Read the model definition and answer for the solid it produces. Units are mm, in the model's axes. A direction names the side the tool comes from. Coordinates: 2 decimals unless noted, no trailing zeros. Order: outer loops, then holes, each group sorted by start corner. A loop starts at its lowest first (then second) coordinate and runs counter-clockwise, first axis right, second up. Notation, with made-up numbers: (2, 62) -> (53, 62) arc R16 cw to (53, 70) -> close; hole circle Ø9 at (-14, -14.5). An arc over 180 degrees is marked (long way). Use CSV: the item, a comma, the result in double quotes.
```python
from build123d import *

# Parameters (mm, degrees)
F0_R     = 12.7
F1_DEPTH = 152.4
F2_R     = 76.19999
F3_R     = 38.1
F4_DEPTH = 41.7364233324
F7_DEPTH = 96.9898923586
F8_DEPTH = 152.401


# Not quite as in the source:
# - a fillet or chamfer is up to 0.001 mm smaller than in the source, because OpenCascade refuses the exact size


with BuildPart() as f1:
    # F0 (on Front) → F1 (new body)
    with BuildSketch(Plane.XZ):
        with BuildLine():
            Line((-39.075684309, -141.72433921), (-39.075684309, 42.0253665879))
            ThreePointArc((-39.075684309, 42.0253665879), (-56.0010235987, 86.8688094558), (-70.825684309, 41.2877726846))
            Line((-70.825684309, 41.2877726846), (-70.825684309, -141.72433921))
            Line((-70.825684309, -141.72433921), (-39.075684309, -141.72433921))
        make_face()
        with Locations((-55.4111076414, 61.47566079)):
            Circle(F0_R, mode=Mode.SUBTRACT)
        with BuildLine():
            Line((-61.300684309, -52.82433921), (-61.300684309, -2.02433921))
            ThreePointArc((-61.300684309, -2.02433921), (-54.950684309, 4.32566079), (-48.600684309, -2.02433921))
            Line((-48.600684309, -2.02433921), (-48.600684309, -52.82433921))
            ThreePointArc((-48.600684309, -52.82433921), (-54.950684309, -59.17433921), (-61.300684309, -52.82433921))
        make_face(mode=Mode.SUBTRACT)
        with BuildLine():
            ThreePointArc((-48.600684309, -2.02433921), (-54.950684309, 4.32566079), (-61.300684309, -2.02433921))
            Line((-61.300684309, -2.02433921), (-61.300684309, -52.82433921))
            ThreePointArc((-61.300684309, -52.82433921), (-54.950684309, -59.17433921), (-48.600684309, -52.82433921))
            Line((-48.600684309, -52.82433921), (-48.600684309, -2.02433921))
        make_face()
    extrude(amount=F1_DEPTH)

    # F2 (radius 76.2 in the source; OpenCascade refuses exactly that, so slightly less here)
    f2_edges = [f1.edges().sort_by_distance(p)[0] for p in [
        (-54.950684, 0, -141.724339),
        (-54.950684, -152.4, -141.724339),
    ]]
    fillet(f2_edges, radius=F2_R)

    # F3 (on face) → F4 (cut, through all)
    with BuildSketch(Plane.YZ.offset(-39.075684309)):
        with Locations((-76.2, -65.52433921)):
            Circle(F3_R)
    extrude(amount=-F4_DEPTH, mode=Mode.SUBTRACT)

    # F6 (on offset) → F7 (cut, through all)
    with BuildSketch(Plane.YZ.offset(-127)):
        Polygon((-24.3093731642, 100.3912016645), (-125.9093731642, 96.466931504), (-125.9093731642, 20.266931504), (-24.3093731642, 20.266931504), align=None)
    extrude(amount=F7_DEPTH, mode=Mode.SUBTRACT)

    # F0 (on Front) → F8 (cut, through all)
    with BuildSketch(Plane.XZ):
        with BuildLine():
            ThreePointArc((-48.600684309, -2.02433921), (-54.950684309, 4.32566079), (-61.300684309, -2.02433921))
            Line((-61.300684309, -2.02433921), (-61.300684309, -52.82433921))
            ThreePointArc((-61.300684309, -52.82433921), (-54.950684309, -59.17433921), (-48.600684309, -52.82433921))
            Line((-48.600684309, -52.82433921), (-48.600684309, -2.02433921))
        make_face()
    extrude(amount=F8_DEPTH, mode=Mode.SUBTRACT)


solid = f1.part
```
Item 1: Straight lines are drawn through the part: line 1 along X through (y, z) = (-20.5, -30.5); line 2 along Y through (x, z) = (-33, 58); line 3 along Z through (x, y) = (-54.5, -76). For each, find the intervals that lie inside material, in ascending order.
Return value:
line 1,"x = -70.83 to -61.3, -48.6 to -39.08"
line 2,"y = -152.4 to -125.91, -24.31 to 0"
line 3,"z = -141.72 to -103.62, 4.31 to 20.27"
Item 2: Find section C-C, the plane x = -64. Give the number of separate pieces and of enclosed holes in the cut face, then the cut area to 3 significant figures.
Return value:
separate pieces,"3"
enclosed holes,"1"
area,"20,000 mm^2"
Item 3: A tool of negligible diameter and unlimited length cuts with its end or side. For faces 4 (the flat face through (-39.076, -92.1, -30.7)), 5 (the flat face through (-56, -24.309, 46)), 6 (the cylindrical face through (-54.728, -22.914, -119.995)), 7 (the flat face through (-61.301, -75, -27)), 8 (the cylindrical face through (-54.73, -84.46, -102.72)), from which of +Z, -Z, +X, -X, +Y, -Y can it reach the whole face along a straight path? Write none if from no direction.
Return value:
face 4,"-Z, +X, +Y, -Y"
face 5,"+Z, +X, -X"
face 6,"-Z, +X, -X, +Y"
face 7,"+Y, -Y"
face 8,"+X, -X"
Item 4: Find section D-D, the plane y = -68.5. Give the vertices of the cut face in (x, z).
Return value:
outline,"(-70.83, -141.33) -> (-39.08, -141.33) -> (-39.08, -102.84) -> (-70.83, -102.84) -> close; (-70.83, -28.21) -> (-61.3, -28.21) -> (-61.3, -2.02) arc R6.35 cw to (-48.6, -2.02) -> (-48.6, -28.21) -> (-39.08, -28.21) -> (-39.08, 20.27) -> (-70.83, 20.27) -> close"
Item 5: Find section B-B, the plane y = -95. Give the vertices of the cut face in (x, z).
Return value:
outline,"(-70.83, -139.37) -> (-39.08, -139.37) -> (-39.08, -98.66) -> (-70.83, -98.66) -> close; (-70.83, -32.39) -> (-61.3, -32.39) -> (-61.3, -2.02) arc R6.35 cw to (-48.6, -2.02) -> (-48.6, -32.39) -> (-39.08, -32.39) -> (-39.08, 20.27) -> (-70.83, 20.27) -> close"
Item 6: The mould has two halves that part along X. Classify faces 1 (the flat face through (-70.826, -92, -29)), 2 (the flat face through (-56, 0, 29)), 3 (the cylindrical face through (-43.68, -11.98, 56.61)): +X half, -X half, draft (parallel to the pull), parting line (faces both ways), or undercut.
Return value:
face 1,"-X half"
face 2,"draft"
face 3,"undercut"
Item 7: Find section A-A, the plane z = -47. Give the vertices of the cut face in (x, y).
Return value:
outline,"(-70.83, -152.4) -> (-61.3, -152.4) -> (-61.3, -109.49) -> (-70.83, -109.49) -> close; (-70.83, -42.91) -> (-61.3, -42.91) -> (-61.3, 0) -> (-70.83, 0) -> close; (-48.6, -152.4) -> (-39.08, -152.4) -> (-39.08, -109.49) -> (-48.6, -109.49) -> close; (-48.6, -42.91) -> (-39.08, -42.91) -> (-39.08, 0) -> (-48.6, 0) -> close"
Item 8: Each of these flat-tipped pins is pushed along its axis until it touches: P1, Ø10, axis at x = -36, y = -55, coming from the -Z side; P2, Ø10, axis at x = -49.5, z = -110, coming from the +Y side; P3, Ø1, axis at x = -67.5, z = 35, coming from the +Y side; P4, Ø1, axis at x = -54.5, y = -21, coming from the -Z side. Where does it stop, or does it pass through?
Return value:
P1,"stops at z = -139.74"
P2,"stops at y = -11.02"
P3,"stops at y = 0"
P4,"stops at z = -118.57"
